Input: dimensioned drawing with shaded views. Units: mm. Origin: part minimum x, y, z. A direction names the side the tool comes from. Coordinates: 2 decimals unless noted, no trailing zeros. Loops run counter-clockwise (first coordinate to the right, second up) from the corner with the lowest first, then second, coordinate; pieces in that order, holes last.
Item 1: Reachability of the marked faces 1 and 2 from +Z, -Z, +X, -X, +Y, -Y: full face, straight path, thin tool, end or side. Return the list, or none.
Item 2: Section query B-B, the plane y = 14.5. Return the cut outline in (x, z), then the cut area to 3 significant figures.
Item 3: Pin query (flat end, axial travel): pin 1 Ø2 at (y, z) = (24, 7.5) entering from -X; pin 2 Ø6 at (x, y) = (41, 28.5) entering from -Z. Return the tip coordinate at first contact, or that it passes through.
Item 4: Section query A-A, the plane x = 200. Return the cut outline in (y, z), then the cut area to 3 significant figures.
Item 5: Line query: probe 1 along Z at (x, y) = (223.5, 25.5); probe 2 along Y at (x, z) = (77, 5.5); probe 3 along Y at (x, z) = (143, 9.75). Output: solid intervals per line, ascending.
Item 6: Section query C-C, the plane z = 7.75. Return the cut outline in (x, y).
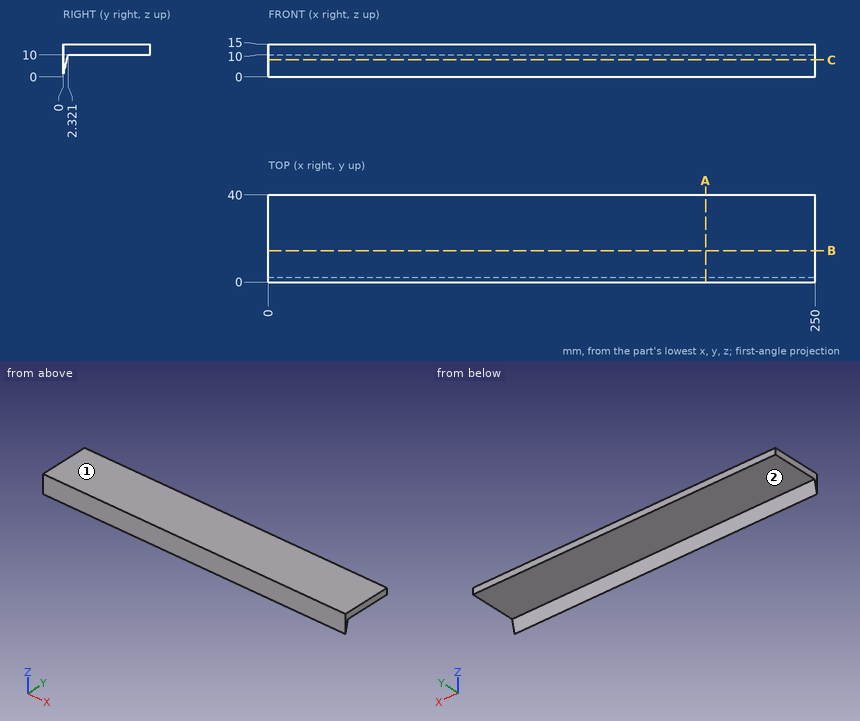
Verdict:
1. face 1: +Z, +X, -X, +Y, -Y
1. face 2: -Z, +X, -X, +Y
2. outline: (0, 10) - (250, 10) - (250, 15) - (0, 15) - close
2. area: 1,250 mm2
3. pin 1: passes through
3. pin 2: stops at z = 10
4. outline: (0, 0) - (2.32, 10) - (40, 10) - (40, 15) - (0, 15) - close
4. area: 212 mm2
5. probe 1: z = 10 to 15
5. probe 2: y = 0 to 1.28
5. probe 3: y = 0 to 2.26
6. outline: (0, 0) - (250, 0) - (250, 1.8) - (0, 1.8) - close
